```python
from build123d import *

# Parameters (mm, degrees)
CHAMFER_1_SIZE           = 1.25
CHAMFER_1_SIZE2          = 0.334936491
SKETCH_2_R               = 2
CUT_EXTRUDE_3_DEPTH      = 1
CUT_EXTRUDE_3_DEPTH_BACK = 8
CHAMFER_2_SIZE           = 1.25
CHAMFER_2_SIZE2          = 0.334936491


with BuildPart() as part:
    # Эскиз1 → Повернуть2 (revolve)
    with BuildSketch(Plane.XY):
        Polygon((0, 0), (25.5, 0), (25.5, 3.5), (3, 3.5), (3, 7), (0, 7), align=None)
    revolve(axis=Axis((0, 7, 0), (0, -1, 0)))

    # Фаска1
    chamfer_1_edges = [part.edges().sort_by_distance(p)[0] for p in [
        (-25.5, 3.5, 0),
    ]]
    chamfer_1_side = [part.faces().sort_by_distance(p)[0] for p in [
        (-24.778751083, 3.5, 0),
    ]]
    chamfer(chamfer_1_edges, length=CHAMFER_1_SIZE, length2=CHAMFER_1_SIZE2, reference=chamfer_1_side[0])

    # Эскиз2 → Вырез-Вытянуть3 (cut, two sides)
    with BuildSketch(Plane(origin=(0, 0, 0), x_dir=(-1, 0, 0), z_dir=(0, -1, 0))) as cut_extrude_3_sk:
        Circle(SKETCH_2_R)
    extrude(amount=CUT_EXTRUDE_3_DEPTH, mode=Mode.SUBTRACT)
    extrude(cut_extrude_3_sk.sketch, amount=-CUT_EXTRUDE_3_DEPTH_BACK, mode=Mode.SUBTRACT)

    # Фаска2
    chamfer_2_edges = [part.edges().sort_by_distance(p)[0] for p in [
        (-25.5, 0, 0),
    ]]
    chamfer_2_side = [part.faces().sort_by_distance(p)[0] for p in [
        (-24.778751083, 0, 0),
    ]]
    chamfer(chamfer_2_edges, length=CHAMFER_2_SIZE, length2=CHAMFER_2_SIZE2, reference=chamfer_2_side[0])


solid = part.part
```
Can you work these out from the model? Positions are in its coordinate system, mm. A direction names the side the tool comes from. Give positions to 0.01 mm unless a question says otherwise; leave off trailing zeros. Write each loop counter-clockwise with the first axis right and the second up, starting at its lowest first coordinate (ties: lowest second). Pieces come first, ordered by that corner, then holes. Notation, with made-up numbers: (74, 51.5) - (105, 51.5) arc R26 ccw to (105, 77.5) - close; hole circle Ø8 at (32, -12.5). An arc over 180 degrees is marked (long way). Write item = value, one per line. Start each with the question number.
1. Imagine slicing it at C-C (y = 2.5). Please give me the cut outline in (x, z).
2. On a 3-axis mill with a long thin cutter (end or side, diameter ignored), from which of +Z, -Z, +X, -X, +Y, -Y can I reach the whole of each face in a straight line? I mean faces 1 (the face through (1, 7, -2)), 2 (the face through (-3, 5, 0)). Say none if no direction works.
3. Thinking about a two-plate mould opening in Z: for faces 3 (the face through (-5.5, 1.8, -24.9)), 4 (the face through (0, 0, -5)), 5 (the face through (0, 3, 2)), which applies, released by +Z, released by -Z, zero draft, split by the parting line, or undercut?
4. For pin 1 (6 mm diameter, centred on x = 5.5, z = -19, fed in from +Y); pin 2 (6.5 mm diameter, centred on x = 0, z = 0, fed in from -Y); pin 3 (3 mm diameter, centred on x = 14.5, y = 2, fed in from -Z), each with a flat end and sliding along its axis, tell me the tip position at first contact or that it passes through.
5. Imagine slicing it at B-B (z = 0). Please give me the cut outline in (x, y).
6. Please list where these lines run through material, in increasing order: line 1 (Z direction, x = 0, y = 4.25); line 2 (Y direction, x = -2, z = -6); line 3 (Z direction, x = -1, y = 1).
7. Imagine slicing it at A-A (x = 0). Please give me the cut outline in (y, z).
Worked answers:
q1.outline = circle Ø51 at (0, 0); hole circle Ø4 at (0, 0)
q2.face_1 = +Z, -Z, +X, -X, +Y
q2.face_2 = +Y
q3.face_3 = split by the parting line
q3.face_4 = zero draft
q3.face_5 = undercut
q4.pin_1 = 3.5
q4.pin_2 = 0
q4.pin_3 = -21.94
q5.outline = (-25.5, 0.33) - (-24.25, 0) - (-2, 0) - (-2, 7) - (-3, 7) - (-3, 3.5) - (-24.25, 3.5) - (-25.5, 3.17) - close; (2, 0) - (24.25, 0) - (25.5, 0.33) - (25.5, 3.17) - (24.25, 3.5) - (3, 3.5) - (3, 7) - (2, 7) - close
q6.line_1 = -3 to -2, 2 to 3
q6.line_2 = 0 to 3.5
q6.line_3 = -25.48 to -1.73, 1.73 to 25.48
q7.outline = (0, -24.25) - (0.33, -25.5) - (3.17, -25.5) - (3.5, -24.25) - (3.5, -3) - (7, -3) - (7, -2) - (0, -2) - close; (0, 2) - (7, 2) - (7, 3) - (3.5, 3) - (3.5, 24.25) - (3.17, 25.5) - (0.33, 25.5) - (0, 24.25) - close
